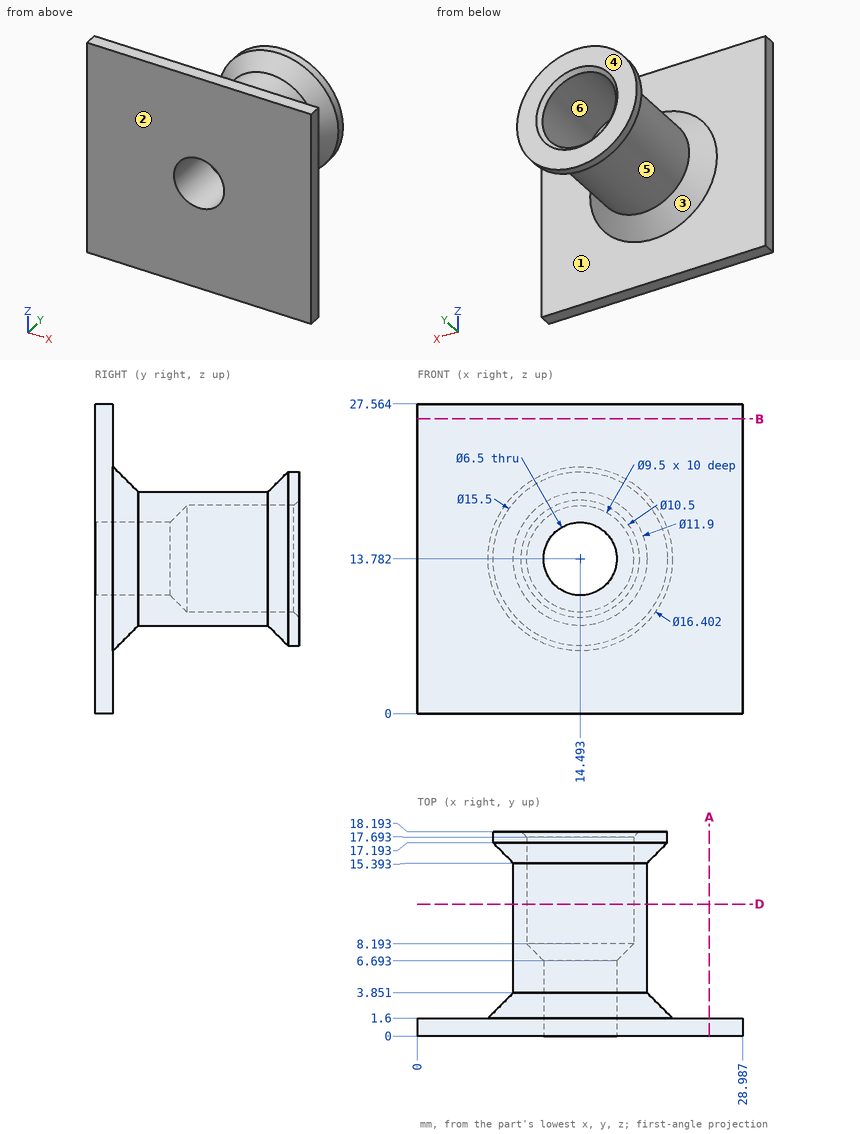
Check sheet for the drawn part. Datum: minimum x, y, z corner. Units: mm. A direction names the side the tool comes from. Round coordinates to 2 decimals unless told otherwise and drop trailing zeros. Order: outer loops, then holes, each group sorted by start corner. A loop starts at its lowest first (then second) coordinate and runs counter-clockwise, first axis right, second up.
(1) Draft check along Y on the marked faces 1, 2 and 3. Enter one of: pulls with the +Y half, pulls with the -Y half, needs draft (parallel to the pull), parting line crosses it, or undercut.
(2) Cross-section at D-D, the plane y = 11.75. Enter the section's corners in (x, z).
(3) Cross-section at A-A, the plane x = 26. Enter the section's corners in (y, z).
(4) Scan lines: probe 1 along X at (y, z) = (1.5, 13.75); probe 2 along X at (y, z) = (15, 13.75); probe 3 along Y at (x, z) = (25.25, 9.5). Record each from-to range of solid material in increasing order.
(5) Cross-section at B-B, the plane z = 26.25. Enter the section's corners in (x, y).
(6) Go/stop test with flat-tipped pins: P1, Ø2, axis at x = 24, y = 15, coming from the +Z side; P2, Ø1.5, axis at x = 19, y = 2.5, coming from the +Z side (1 decimal); P3, Ø6, axis at y = 8.5, z = 16, coming from the +X side; P4, Ø3, axis at x = 17, y = 9, coming from the -Z side. Record where each tip stops, or that it passes through.
(7) Access from +Z, -Z, +X, -X, +Y, -Y to the whole of each face (thin tool, end or side, straight path). Record for the marked faces 4, 5 and 6.
Check sheet entries:
1. face 1: pulls with the +Y half
1. face 2: pulls with the -Y half
1. face 3: undercut
2. outline: circle Ø11.9 at (14.49, 13.78); hole circle Ø9.5 at (14.49, 13.78)
3. outline: (0, 0) - (1.6, 0) - (1.6, 27.56) - (0, 27.56) - close
4. probe 1: x = 0 to 11.24, 17.74 to 28.99
4. probe 2: x = 8.54 to 9.74, 19.24 to 20.44
4. probe 3: y = 0 to 1.6
5. outline: (0, 0) - (28.99, 0) - (28.99, 1.6) - (0, 1.6) - close
6. P1: passes through
6. P2: stops at z = 20.6
6. P3: stops at x = 20.44
6. P4: stops at z = 7.92
7. face 4: +Z, -Z, +X, -X, +Y
7. face 5: none
7. face 6: +Y
